Source: three-view drawing plus pictorial views. Frame: mm from the lowest corner of the part. Give positions to 0.01 mm unless a question says otherwise; leave off trailing zeros. Order: outer loops, then holes, each group sorted by start corner. A loop starts at its lowest first (then second) coordinate and runs counter-clockwise, first axis right, second up. Notation, with made-up numbers: (0.5, 75.25) -> (53.5, 75.25) arc R18 cw to (53.5, 82.25) -> close; hole circle Ø6 at (25, -29.75). An arc over 180 degrees is marked (long way). Write item = value, one per line.
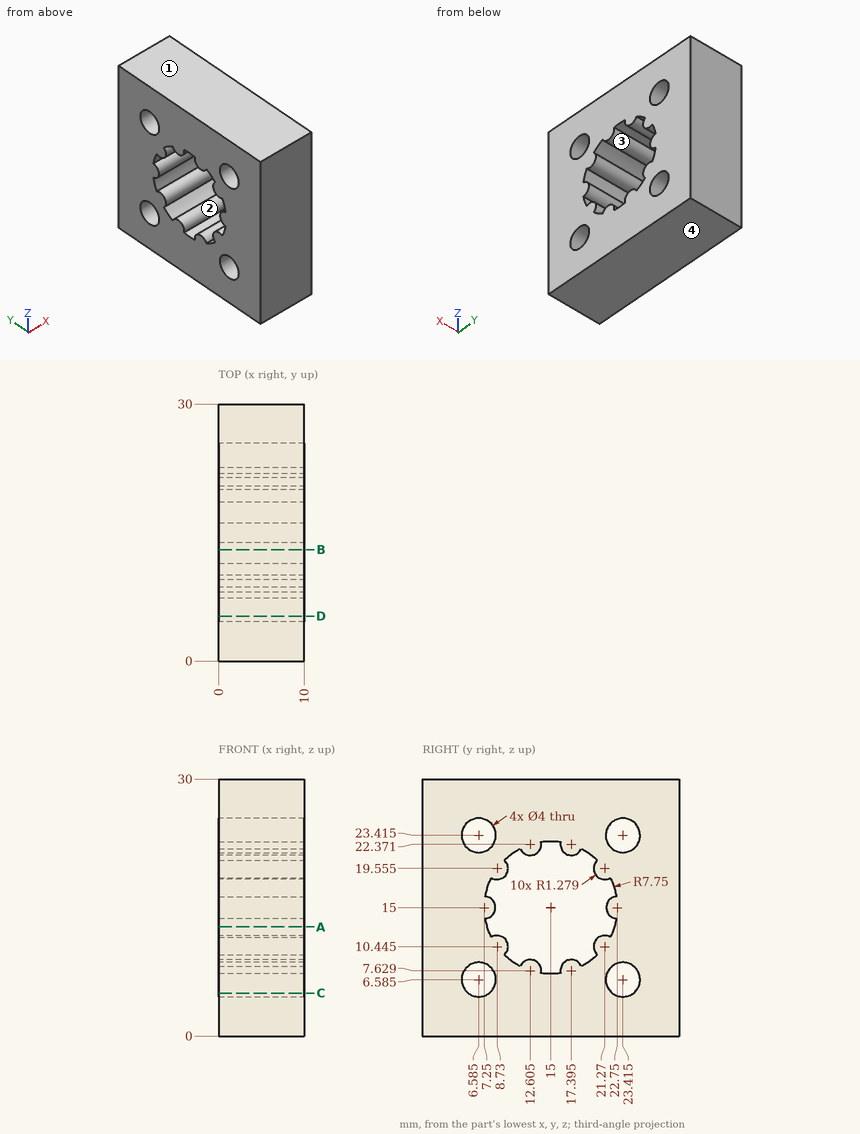
1) Section query D-D (y = 5.25). Output: boundary loops of the cut face in (x, z) (1 decimal).
Check sheet entries:
outline = (0, 0) -> (10, 0) -> (10, 5.1) -> (0, 5.1) -> close; (0, 8.1) -> (10, 8.1) -> (10, 21.9) -> (0, 21.9) -> close; (0, 24.9) -> (10, 24.9) -> (10, 30) -> (0, 30) -> close
2) Line query: line 1 (Y direction, x = 3.75, z = 5.25) (1 decimal); line 2 (Y direction, x = 8.25, z = 23.25); line 3 (Z direction, x = 0.5, y = 4.75) (1 decimal). Output: solid intervals per line, ascending. Write a range as from..to.
Check sheet entries:
line_1 = 0..5.1, 8.1..21.9, 24.9..30
line_2 = 0..4.59, 8.58..21.42, 25.41..30
line_3 = 0..5.8, 7.4..22.6, 24.2..30
3) Section query A-A (z = 12.75). Output: boundary loops of the cut face in (x, y).
Check sheet entries:
outline = (0, 0) -> (10, 0) -> (10, 7.58) -> (0, 7.58) -> close; (0, 22.42) -> (10, 22.42) -> (10, 30) -> (0, 30) -> close
4) Section query B-B (y = 13). Output: boundary loops of the cut face in (x, z) (1 decimal), plus the area to 3 significant figures.
Check sheet entries:
outline = (0, 0) -> (10, 0) -> (10, 8.8) -> (0, 8.8) -> close; (0, 21.2) -> (10, 21.2) -> (10, 30) -> (0, 30) -> close
area = 177 mm²
5) Section query C-C (z = 5). Output: boundary loops of the cut face in (x, y) (1 decimal), plus the area to 3 significant figures.
Check sheet entries:
outline = (0, 0) -> (10, 0) -> (10, 5.4) -> (0, 5.4) -> close; (0, 7.8) -> (10, 7.8) -> (10, 22.2) -> (0, 22.2) -> close; (0, 24.6) -> (10, 24.6) -> (10, 30) -> (0, 30) -> close
area = 251 mm²
6) Mould query, pull axis Z, two halves, no side actions, for the marked faces 1, 2, 3 and 4. Classes: +Z half, -Z half, draft (parallel to the pull), parting line (faces both ways), or undercut.
Check sheet entries:
face_1 = +Z half
face_2 = undercut
face_3 = undercut
face_4 = -Z half
7) First-contact query: P1, Ø3, axis at y = 23.41, z = 23.41, coming from the +X side. Flat tip, straight axial feed; report the tip coordinate or a pass-through.
Check sheet entries:
P1 = through
